Design review of the part built by this model. Coordinates are the model's own, in mm. A direction names the side the tool comes from. Coordinates: 2 decimals unless noted, no trailing zeros. Write each loop counter-clockwise with the first axis right and the second up, starting at its lowest first coordinate (ties: lowest second). Pieces come first, ordered by that corner, then holes.
Q1. Add section B-B, the plane z = 3.77. Give the boundary of the cut face in (x, y).
Q2. Add section A-A, the plane y = 3. Give the number of separate pieces and of enclosed holes in the cut face, plus the area to 3 significant figures.
Q3. Machinability: for faces 1 (the face through (-1, 0, 15)), 2 (the face through (-6.354, 10.437, 3.239)), 3 (the face through (-8, 8.05, 4)), which of the approach directions +Z, -Z, +X, -X, +Y, -Y give a long, thin tool a straight path to every point of the face, cutting with its end or side? Answer none if there is none.
Q4. Add section C-C, the plane x = -15. Give the boundary of the cut face in (y, z).
Q5. To check wall thickness, follow probe 1 along X at (y, z) = (9, 3.77); probe 2 along X at (y, z) = (6, 11.5); probe 3 along X at (y, z) = (5.25, 15.5). State the ranges of each line that lie inside material, in increasing order.
Q6. Clearance check with flat-ended pins moving along their axes: pin 1 Ø0.5 at (x, z) = (-7, 6.5) entering from -Y; pin 2 Ø3 at (x, z) = (-7.925, 15.925) entering from -Y; pin 3 Ø1.7 at (x, z) = (-7.5, 4) entering from -Y; pin 4 Ø4 at (x, z) = (-7.92, 23.89) entering from -Y. State where each tip first meets the part, or that it passes through.
Q7. Add section D-D, the plane z = 22.5. Give the boundary of the cut face in (x, y), plus the area to 3 significant figures.
from build123d import *

# Parameters (mm, degrees)
BOSS_EXTRUDE1_DEPTH = 15.85
SKETCH3_R           = 2.45
BOSS_EXTRUDE2_DEPTH = 1.8
SHELL1_T            = -1.5
BOSS_EXTRUDE3_REACH = 39.343
SKETCH4_R           = 3.25
SKETCH4_R_2         = 2.45


with BuildPart() as part:
    # Sketch2 → Boss-Extrude1 (new body)
    with BuildSketch(Plane(origin=(0, 0, 0), x_dir=(0, 0, -1), z_dir=(1, 0, 0))):
        Polygon((0, 0), (-31.85, 0), (-31.85, 1.8), (-7.54, 9.55), (0, 9.55), align=None)
    extrude(amount=-BOSS_EXTRUDE1_DEPTH)

    # Sketch3 → Boss-Extrude2 (add)
    with BuildSketch(Plane(origin=(0, 9.55, 0), x_dir=(1, 0, 0), z_dir=(0, 1, 0))):
        with Locations(Location((-11.8875, -3.77, 0), (0, 0, 270))):
            Circle(SKETCH3_R)
        with Locations(Location((-3.9625, -3.77, 0), (0, 0, 270))):
            Circle(SKETCH3_R)
    extrude(amount=BOSS_EXTRUDE2_DEPTH)

    # Shell1
    shell1_openings = [part.faces().sort_by_distance(p)[0] for p in [
        (-7.925, 0, 15.925),
    ]]
    offset(amount=SHELL1_T, openings=shell1_openings, kind=Kind.INTERSECTION)

    # Boss-Extrude3: up to this plane
    boss_extrude3_end = Plane(origin=(-15.85, 0.370866339, 31.394393835), z_dir=(0, 0.952755774285987, 0.30373744346838355))
    # Sketch4 → Boss-Extrude3 (add, up to the surface)
    with BuildSketch(Plane(origin=(0, 0, 0), x_dir=(1, 0, 0), z_dir=(0, 1, 0)), mode=Mode.PRIVATE) as boss_extrude3_sk1:
        with Locations(Location((-7.925, -23.8875, 0), (0, 0, 270))):
            Circle(SKETCH4_R)
        with Locations(Location((-7.925, -23.8875, 0), (0, 0, 270))):
            Circle(SKETCH4_R_2, mode=Mode.SUBTRACT)
    boss_extrude3_tool1 = split(extrude(boss_extrude3_sk1.sketch, amount=BOSS_EXTRUDE3_REACH, mode=Mode.PRIVATE), bisect_by=boss_extrude3_end, keep=Keep.BOTH, mode=Mode.PRIVATE)
    add(boss_extrude3_tool1.solids().sort_by_distance((-7.925, 0, 20.729424))[0])
    # Sketch4 → Boss-Extrude3 (add, up to the surface)
    with BuildSketch(Plane(origin=(0, 0, 0), x_dir=(1, 0, 0), z_dir=(0, 1, 0)), mode=Mode.PRIVATE) as boss_extrude3_sk2:
        with Locations(Location((-7.925, -15.925, 0), (0, 0, 270))):
            Circle(SKETCH4_R)
        with Locations(Location((-7.925, -15.925, 0), (0, 0, 270))):
            Circle(SKETCH4_R_2, mode=Mode.SUBTRACT)
    boss_extrude3_tool2 = split(extrude(boss_extrude3_sk2.sketch, amount=BOSS_EXTRUDE3_REACH, mode=Mode.PRIVATE), bisect_by=boss_extrude3_end, keep=Keep.BOTH, mode=Mode.PRIVATE)
    add(boss_extrude3_tool2.solids().sort_by_distance((-7.925, 0, 12.766924))[0])
    # Sketch4 → Boss-Extrude3 (add, up to the surface)
    with BuildSketch(Plane(origin=(0, 0, 0), x_dir=(1, 0, 0), z_dir=(0, 1, 0)), mode=Mode.PRIVATE) as boss_extrude3_sk3:
        with Locations(Location((-7.925, -7.9625, 0), (0, 0, 11.641598249))):
            Circle(SKETCH4_R)
        with Locations(Location((-7.925, -7.9625, 0), (0, 0, 15.526222554))):
            Circle(SKETCH4_R_2, mode=Mode.SUBTRACT)
    boss_extrude3_tool3 = split(extrude(boss_extrude3_sk3.sketch, amount=BOSS_EXTRUDE3_REACH, mode=Mode.PRIVATE), bisect_by=boss_extrude3_end, keep=Keep.BOTH, mode=Mode.PRIVATE)
    add(boss_extrude3_tool3.solids().sort_by_distance((-11.018111, 0, 8.599765))[0])


solid = part.part
Here are the results:
1. outline: (-15.85, 0) - (-14.35, 0) - (-14.35, 8.05) - (-12.84, 8.05) - (-12.84, 9.85) - (-10.94, 9.85) - (-10.94, 8.05) - (-4.91, 8.05) - (-4.91, 9.85) - (-3.01, 9.85) - (-3.01, 8.05) - (-1.5, 8.05) - (-1.5, 0) - (0, 0) - (0, 9.55) - (-1.51, 9.55) - (-1.51, 11.35) - (-6.41, 11.35) - (-6.41, 9.55) - (-9.44, 9.55) - (-9.44, 11.35) - (-14.34, 11.35) - (-14.34, 9.55) - (-15.85, 9.55) - close
2. separate pieces: 3
2. enclosed holes: 4
2. area: 202 mm2
3. face 1: +Z, -Z, +X, -X, -Y
3. face 2: +Y
3. face 3: -Y
4. outline: (0, 0) - (9.55, 0) - (9.55, 7.54) - (1.8, 31.85) - (0, 31.85) - close
5. probe 1: x = -15.85 to -12.84, -10.94 to -4.91, -3.01 to 0
5. probe 2: x = -15.85 to -14.35, -1.5 to 0
5. probe 3: x = -15.85 to -14.35, -11.15 to -10.34, -5.51 to -4.7, -1.5 to 0
6. pin 1: stops at y = 8.05
6. pin 2: stops at y = 4.82
6. pin 3: stops at y = 0
6. pin 4: stops at y = 2.13
7. outline: (-15.85, 0) - (-14.35, 0) - (-14.35, 3.21) - (-10.86, 3.21) - (-10.86, 0) - (-9.94, 0) - (-9.94, 3.21) - (-5.91, 3.21) - (-5.91, 0) - (-4.99, 0) - (-4.99, 3.21) - (-1.5, 3.21) - (-1.5, 0) - (0, 0) - (0, 4.78) - (-15.85, 4.78) - close
7. area: 40.5 mm2
